from build123d import *

# Parameters (mm, degrees)
F0_R     = 12.065
F0_R_2   = 6.35
F1_DEPTH = 6.35
F2_R     = 2.06375
F3_DEPTH = 14.883615
F4_R     = 2.06375
F5_DEPTH = 14.883615


with BuildPart() as f1:
    # F0 (on Top) → F1 (new body)
    with BuildSketch(Plane.XY):
        with BuildLine():
            Line((-35.814, 15.067575), (-50.881575, 17.353575))
            Line((-50.881575, 17.353575), (-51.357825, 14.214497))
            Line((-51.357825, 14.214497), (-53.167575, 2.286))
            ThreePointArc((-53.167575, 2.286), (-47.137938, 12.27083), (-35.814, 15.067575))
        make_face()
        Polygon((-51.357825, 14.214497), (-50.881575, 17.353575), (-59.043177, 18.591825), (-59.519427, 15.452747), align=None)
        with BuildLine():
            Line((10.845984, 7.988484), (-35.814, 15.067575))
            ThreePointArc((-35.814, 15.067575), (-47.137938, 12.27083), (-53.167575, 2.286))
            ThreePointArc((-53.167575, 2.286), (-48.876307, -10.776307), (-35.814, -15.067575))
            Line((-35.814, -15.067575), (1.42875, -9.417234))
            ThreePointArc((1.42875, -9.417234), (6.735192, -6.735192), (9.417234, -1.42875))
            Line((9.417234, -1.42875), (10.369734, 4.849406))
            Line((10.369734, 4.849406), (10.845984, 7.988484))
        make_face()
        with Locations((-38.1, 0)):
            Circle(F0_R, mode=Mode.SUBTRACT)
        with BuildLine():
            Line((-27.084666, 10.531857), (-6.066692, 7.343083))
            ThreePointArc((-6.066692, 7.343083), (-9.525, 0), (-6.066692, -7.343083))
            Line((-6.066692, -7.343083), (-27.084666, -10.531857))
            ThreePointArc((-27.084666, -10.531857), (-22.86, 0), (-27.084666, 10.531857))
        make_face(mode=Mode.SUBTRACT)
        Circle(F0_R_2, mode=Mode.SUBTRACT)
        Polygon((19.007587, 6.750234), (10.845984, 7.988484), (10.369734, 4.849406), (18.531337, 3.611156), align=None)
    extrude(amount=F1_DEPTH)

    # F2 (on face) → F3 (cut, through all)
    with BuildSketch(Plane(origin=(0.9525, 6.278156, 0), x_dir=(0.988686, -0.15, 0), z_dir=(-0.15, -0.988686, 0))):
        with Locations((-57.036436, 3.175)):
            Circle(F2_R)
    extrude(amount=-F3_DEPTH, mode=Mode.SUBTRACT)

    # F4 (on face) → F5 (cut, through all)
    with BuildSketch(Plane(origin=(0.9525, 6.278156, 0), x_dir=(0.988686, -0.15, 0), z_dir=(-0.15, -0.988686, 0))):
        with Locations((13.6525, 3.175)):
            Circle(F4_R)
    extrude(amount=-F5_DEPTH, mode=Mode.SUBTRACT)


solid = f1.part
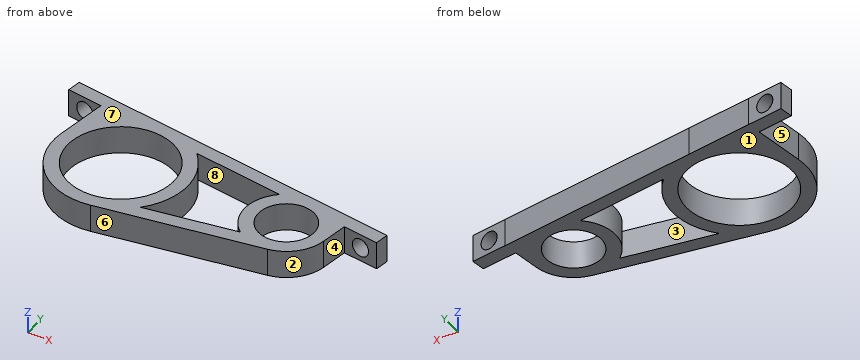
Verification items for the finished model (mm, model axes). Face numbers are marked on the shaded views. A direction names the side the tool comes from. Coordinates: 2 decimals unless noted, no trailing zeros. Order: outer loops, then holes, each group sorted by start corner. A loop starts at its lowest first (then second) coordinate and runs counter-clockwise, first axis right, second up. Notation, with made-up numbers: M -0.5,-20 L 39.5,-20 A27 cw 39.5,12 Z; hole C 61,45 d6. An arc over 180 degrees is marked long. One line per item, written item: value. Start each with the question number.
Item 1: Sectioned sample at C-C (y = -4.5). Enter the section's corners in (x, z).
Item 2: Sectioned sample at B-B (x = 5). Enter the section's corners in (y, z).
Item 3: Sectioned sample at D-D (x = -7.5). Enter the section's corners in (y, z).
Item 4: Scan lines: probe 1 along X at (y, z) = (4.5, 3); probe 2 along X at (y, z) = (5, 3.25); probe 3 along Y at (x, z) = (-38.1, 4.5) (3 decimals). Record each from-to range of solid material in increasing order.
Item 5: Gauge pin test, flat ends, axial feed: pin 1 (3 mm diameter, centred on x = -28.5, y = -5.5, fed in from +Z); pin 2 (3 mm diameter, centred on x = -30, z = 5.5, fed in from -Y); pin 3 (3 mm diameter, centred on x = 5, z = 2.5, fed in from +Y); pin 4 (1.5 mm diameter, centred on y = -8, z = 4.5, fed in from -X). Record the tip position at first contact, or that the pin passes through.
Item 6: Mould release check, pull along Y, two halves, no side actions. Record for the marked faces 6, 7 and 8: released by +Y, released by -Y, zero draft, split by the parting line, or undercut.
Item 7: Access from +Z, -Z, +X, -X, +Y, -Y to the whole of each face (thin tool, end or side, straight path). Record for the marked faces 1, 2, 3, 4 and 5.
Item 8: Sectioned sample at A-A (z = 4). Count the separate pieces of the cut face and the enclosed holes in it, then the cut area to 3 significant figures.
Conclusion:
1. outline: M -52.66,0 L -49.29,0 L -49.29,6.35 L -52.66,6.35 Z; M -26.91,0 L -23.54,0 L -23.54,6.35 L -26.91,6.35 Z; M -8.39,0 L -4.48,0 L -4.48,6.35 L -8.39,6.35 Z; M 4.48,0 L 8.39,0 L 8.39,6.35 L 4.48,6.35 Z
2. outline: M -8.11,0 L -3.91,0 L -3.91,6.35 L -8.11,6.35 Z; M 3.91,0 L 8.88,0 L 8.88,6.35 L 3.91,6.35 Z
3. outline: M -10.77,0 L -7.56,0 L -7.56,6.35 L -10.77,6.35 Z; M -5.87,0 L 5.87,0 L 5.87,6.35 L -5.87,6.35 Z; M 7.56,0 L 10.77,0 L 10.77,6.35 L 7.56,6.35 Z
4. probe 1: x = -52.83 to -49.29, -26.91 to -23.54, -8.39 to -4.48, 4.48 to 10.32, 16.57 to 18.67
4. probe 2: x = -52.76 to -49.08, -27.12 to -23.7, -8.11 to -3.91, 3.91 to 12.48, 16.65 to 18.74
4. probe 3: y = -15.24 to -12.065, 12.065 to 15.414
5. pin 1: stops at z = 6.35
5. pin 2: stops at y = -14.41
5. pin 3: stops at y = 9.1
5. pin 4: stops at x = -51.51
6. face 6: released by -Y
6. face 7: zero draft
6. face 8: undercut
7. face 1: -Z, +X, -X, +Y, -Y
7. face 2: +Z, -Z, +X, -Y
7. face 3: +Z, -Z
7. face 4: +Z, -Z, -Y
7. face 5: +Z, -Z, -X
8. separate pieces: 3
8. enclosed holes: 3
8. area: 696 mm^2
